from build123d import *

# Parameters (mm, degrees)
SKETCH_1_R           = 1.5
EXTRUDE_1_DEPTH      = 6
EXTRUDE_2_DEPTH      = 15
HOLE_WIZARD_41_D     = 3.048
HOLE_WIZARD_41_DEPTH = 6
HOLE_WIZARD_41_TIP   = 0.915711583


with BuildPart() as part:
    # Эскиз1 → Бобышка-Вытянуть1 (new body)
    with BuildSketch(Plane(origin=(0, 0, 0), x_dir=(1, 0, 0), z_dir=(0, 1, 0))):
        with Locations(Location((0, 0, 0), (0, 0, 270))):
            Circle(SKETCH_1_R)
    extrude(amount=EXTRUDE_1_DEPTH)

    # Эскиз2 → Бобышка-Вытянуть2 (add)
    with BuildSketch(Plane(origin=(0, 6, 0), x_dir=(1, 0, 0), z_dir=(0, 1, 0))):
        Polygon((2.75, 0), (1.375, 2.38156986), (-1.375, 2.38156986), (-2.75, 0), (-1.375, -2.38156986), (1.375, -2.38156986), align=None)
    extrude(amount=EXTRUDE_2_DEPTH)

    # Сверло под метчик  спиральное #41
    with Locations(Plane(origin=(0, 21, 0), x_dir=(1, 0, 0), z_dir=(0, 1, 0))):
        with Locations((0, 0)):
            Hole(HOLE_WIZARD_41_D / 2, depth=HOLE_WIZARD_41_DEPTH)
            with Locations((0, 0, -(HOLE_WIZARD_41_DEPTH + HOLE_WIZARD_41_TIP / 2))):  # 118° drill point
                Cone(0, HOLE_WIZARD_41_D / 2, HOLE_WIZARD_41_TIP, mode=Mode.SUBTRACT)


solid = part.part
Read the model definition and answer for the solid it produces. Units are mm, in the model's axes. A direction names the side the tool comes from. Round coordinates to 2 decimals unless told otherwise and drop trailing zeros. Write each loop counter-clockwise with the first axis right and the second up, starting at its lowest first coordinate (ties: lowest second). Pieces come first, ordered by that corner, then holes.
Q1. Find section B-B on y = 11.25. Determine the outline of the cut face in (x, z) (3 decimals).
Values:
outline: (-2.75, 0) - (-1.375, -2.382) - (1.375, -2.382) - (2.75, 0) - (1.375, 2.382) - (-1.375, 2.382) - close
Q2. Straight lines are drawn through the part: line 1 (Z direction, x = 0, y = 18.2); line 2 (Y direction, x = 1.3, z = 1.15); line 3 (Z direction, x = -0.1, y = 14.25). For each, find the intervals that lie inside material, in ascending order.
Values:
line 1: z = -2.38 to -1.52, 1.52 to 2.38
line 2: y = 6 to 21
line 3: z = -2.38 to -0.26, 0.26 to 2.38
Q3. A tool of negligible diameter and unlimited length cuts with its end or side. For faces 1 (the face through (0.45, 2.96, 1.43)), 2 (the face through (0, 0, 0)), 3 (the face through (0.2, 17.96, -1.51)), from which of +Z, -Z, +X, -X, +Y, -Y can it reach the whole face along a straight path? Write none if from no direction.
Values:
face 1: -Y
face 2: +Z, -Z, +X, -X, -Y
face 3: +Y
Q4. Find section A-A on y = 19. Determine the outline of the cut face in (x, z) (3 decimals).
Values:
outline: (-2.75, 0) - (-1.375, -2.382) - (1.375, -2.382) - (2.75, 0) - (1.375, 2.382) - (-1.375, 2.382) - close; hole circle Ø3.048 at (0, 0)
Q5. Find section C-C on x = 1.75. Determine the outline of the cut face in (y, z).
Values:
outline: (6, -1.73) - (21, -1.73) - (21, 1.73) - (6, 1.73) - close
Q6. The mould has two halves that part along Z. Classify faces 4 (the face through (-2.05, 13.4, -1.21)), 5 (the face through (-0.21, 14.243, 0.161)), 6 (the face through (0, 6, -2)): released by +Z, released by -Z, zero draft, split by the parting line, or undercut.
Values:
face 4: released by -Z
face 5: undercut
face 6: zero draft
